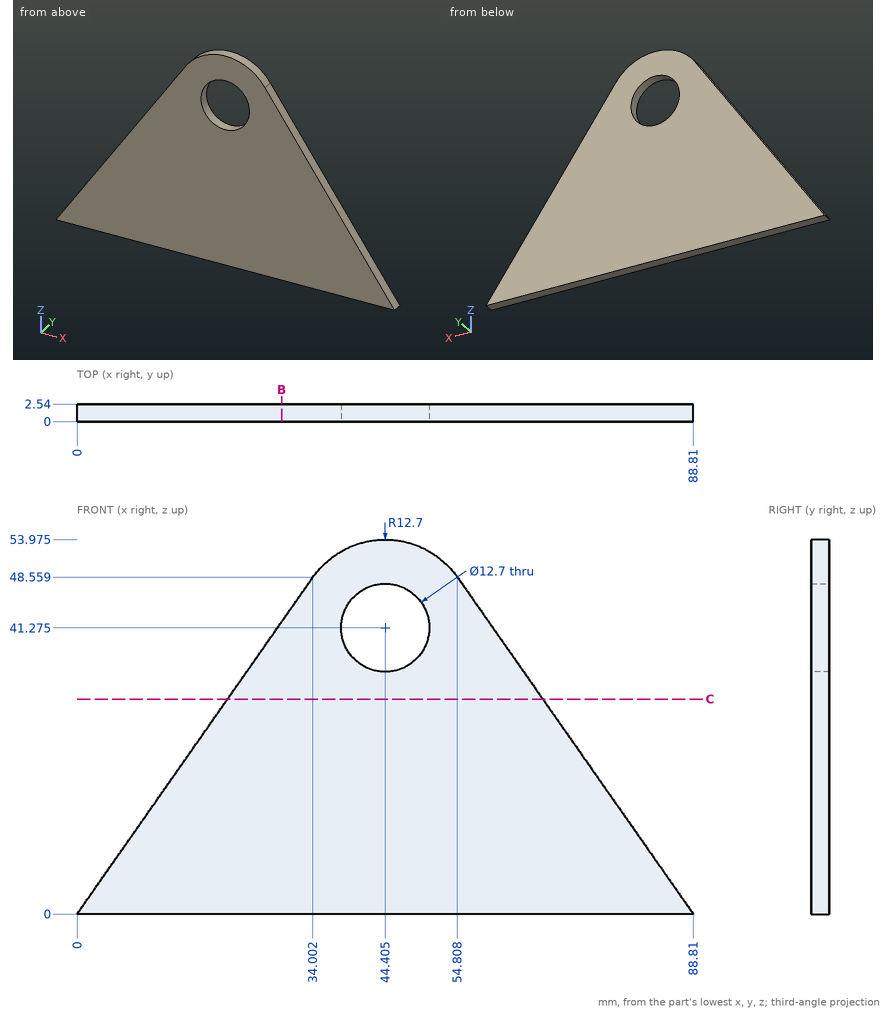
For this review, use the dimensioned drawing (mm, ordinates from the lowest corner) and the shaded views. Round coordinates to 2 decimals unless told otherwise and drop trailing zeros. Write each loop counter-clockwise with the first axis right and the second up, starting at its lowest first coordinate (ties: lowest second). Pieces come first, ordered by that corner, then holes. Notation, with made-up numbers: (62.25, -40) -> (83.25, -40) arc R19 cw to (83.25, -5) -> close; hole circle Ø9 at (-29.5, 59.25). An arc over 180 degrees is marked (long way). Use CSV: the item, a comma, the result in double quotes.
Q1. Consider section C-C (z = 31). Give the boundary of the cut face in (x, y).
Checks:
outline,"(21.71, 0) -> (67.1, 0) -> (67.1, 2.54) -> (21.71, 2.54) -> close"
Q2. For pin 1 Ø8 at (x, z) = (19, 40) entering from +Y; pin 2 Ø1 at (y, z) = (1.5, 48) entering from +X, all flat-tipped, find the tip position at first contact; note any pin that passes through.
Checks:
pin 1,"through"
pin 2,"x = 55.55"
Q3. To check wall thickness, follow probe 1 along X at (y, z) = (1.9, 39) (1 decimal); probe 2 along Z at (x, y) = (65, 1.4) (1 decimal); probe 3 along X at (y, z) = (1.2, 19) (1 decimal). State the ranges of each line that lie inside material, in increasing order. Write a range as [from, to].
Checks:
probe 1,"[27.3, 38.5], [50.3, 61.5]"
probe 2,"[0, 34]"
probe 3,"[13.3, 75.5]"
Q4. Consider section B-B (x = 29.5). Give the boundary of the cut face in (y, z), then the cut area to 3 significant figures.
Checks:
outline,"(0, 0) -> (2.54, 0) -> (2.54, 42.13) -> (0, 42.13) -> close"
area,"107 mm²"
